Work out the finished part from the listing and answer in its coordinate system (mm). A direction names the side the tool comes from. Coordinates: 2 decimals unless noted, no trailing zeros. Write each loop counter-clockwise with the first axis right and the second up, starting at its lowest first coordinate (ties: lowest second). Pieces come first, ordered by that corner, then holes. Notation, with made-up numbers: M 17,23 L 63,23 A5 ccw 63,30 Z; hole C -27,-10.75 d3. An arc over 180 degrees is marked long. Answer as CSV lines item,"result". Start each with the question number.
(1) The mould has two halves that part along Z. Classify faces 3 (the cylindrical face through (-0.59, 4.46, 12.32)), 4 (the cylindrical face through (-6, 0, 26)), 5 (the flat face through (0, 0, 27)): released by +Z, released by -Z, zero draft, split by the parting line, or undercut.
(2) Find the intervals of material crossed by L1, parallel to Z at x = 3.5, y = 4.5; L2, parallel to Y at x = 0.25, z = 17; L3, parallel to Y at x = 3.5, z = 1.25, in increasing order. Write a range as [from, to].
(3) A cutting plane is placed at A-A on y = 0. Give the vertices of the cut face in (x, z).
(4) For faces 1 (the flat face through (-1.4, 4.5, 0)), 2 (the flat face through (0, 0, -2)), determine the directions among +Z, -Z, +X, -X, +Y, -Y from which every point of the face is accessible in a straight line to the end or side of a thin tool.
(5) Flat-ended cylindrical pins translate along their axes: P1, Ø2, axis at x = -3, z = 23, coming from the -Y side; P2, Ø5, axis at x = -3.5, z = 19, coming from the -Y side; P3, Ø2, axis at y = 0, z = 8, coming from the -X side. Find the tip coordinate at first contact, or state that the pin passes through.
(6) A cutting plane is placed at C-C on z = 14.25. Give the vertices of the cut face in (x, y).
from build123d import *

# Parameters (mm, degrees)
SKETCH1_R           = 4.5
BOSS_EXTRUDE1_DEPTH = 25
SKETCH2_R           = 6
BOSS_EXTRUDE2_DEPTH = 2
SKETCH3_R           = 6
BOSS_EXTRUDE3_DEPTH = 2


with BuildPart() as part:
    # Sketch1 → Boss-Extrude1 (new body)
    with BuildSketch(Plane.XY):
        Circle(SKETCH1_R)
    extrude(amount=BOSS_EXTRUDE1_DEPTH)

    # Sketch2 → Boss-Extrude2 (add)
    with BuildSketch(Plane.XY):
        Circle(SKETCH2_R)
    extrude(amount=-BOSS_EXTRUDE2_DEPTH)

    # Sketch3 → Boss-Extrude3 (add)
    with BuildSketch(Plane.XY.offset(25)):
        Circle(SKETCH3_R)
    extrude(amount=BOSS_EXTRUDE3_DEPTH)


solid = part.part
Here are the results:
1,face 3,"undercut"
1,face 4,"zero draft"
1,face 5,"released by +Z"
2,L1,"z = [-2, 0], [25, 27]"
2,L2,"y = [-4.49, 4.49]"
2,L3,"y = [-2.83, 2.83]"
3,outline,"M -6,-2 L 6,-2 L 6,0 L 4.5,0 L 4.5,25 L 6,25 L 6,27 L -6,27 L -6,25 L -4.5,25 L -4.5,0 L -6,0 Z"
4,face 1,"none"
4,face 2,"-Z, +X, -X, +Y, -Y"
5,P1,"stops at y = -4.03"
5,P2,"stops at y = -4.39"
5,P3,"stops at x = -4.5"
6,outline,"C 0,0 d9"
